Can you work these out from the model? Positions are in its coordinate system, mm. A direction names the side the tool comes from. Round coordinates to 2 decimals unless told otherwise and drop trailing zeros. Loops run counter-clockwise (first coordinate to the right, second up) from the corner with the lowest first, then second, coordinate; pieces in that order, holes last. Notation, with made-up numbers: (-37, 41.25) -> (-15, 41.25) arc R27 ccw to (-15, 78.25) -> close; hole circle Ø8 at (-27, 40). An arc over 180 degrees is marked (long way). Use a Markdown table: item, result.
from build123d import *

# Parameters (mm, degrees)
F0_R      = 1.5
F1_DEPTH  = 1
F2_W      = 1
F2_H      = 30
F3_DEPTH  = 5
F4_W      = 1
F4_H      = 30
F5_DEPTH  = 5
F6_R      = 0.5
F7_DEPTH  = 25
F9_DEPTH  = 25
F10_W     = 5
F10_H     = 35
F11_DEPTH = 25
F12_R     = 1.5
F13_DEPTH = 25


with BuildPart() as f1:
    # F0 (on Right) → F1 (new body)
    with BuildSketch(Plane.YZ):
        with BuildLine():
            Line((-6, 17), (-11, 17))
            Line((-11, 17), (-11, 0))
            Line((-11, 0), (-11, -17))
            Line((-11, -17), (-6, -17))
            Line((-6, -17), (-6, -15))
            Line((-6, -15), (-1.664101, -8.496151))
            ThreePointArc((-1.664101, -8.496151), (0, -7.605551), (1.664101, -8.496151))
            Line((1.664101, -8.496151), (6, -15))
            Line((6, -15), (6, -17))
            Line((6, -17), (11, -17))
            Line((11, -17), (11, 0))
            Line((11, 0), (11, 17))
            Line((11, 17), (6, 17))
            Line((6, 17), (6, 15))
            Line((6, 15), (1.664101, 8.496151))
            ThreePointArc((1.664101, 8.496151), (0, 7.605551), (-1.664101, 8.496151))
            Line((-1.664101, 8.496151), (-6, 15))
            Line((-6, 15), (-6, 17))
        make_face()
        with Locations((-2, 0)):
            Circle(F0_R, mode=Mode.SUBTRACT)
        with Locations((2, 0)):
            Circle(F0_R, mode=Mode.SUBTRACT)
    extrude(amount=F1_DEPTH)

    # F2 (on face) → F3 (join)
    with BuildSketch(Plane.XZ.offset(11)):
        with Locations((0.5, 0)):
            Rectangle(F2_W, F2_H)
    extrude(amount=F3_DEPTH)

    # F4 (on face) → F5 (join)
    with BuildSketch(Plane(origin=(0, 11, 0), x_dir=(-1, 0, 0), z_dir=(0, 1, 0))):
        with Locations((-0.5, 0)):
            Rectangle(F4_W, F4_H)
    extrude(amount=F5_DEPTH)

    # F6 (on face) → F7 (cut)
    with BuildSketch(Plane.YZ.offset(1)):
        with Locations((-11.5, 15)):
            Circle(F6_R)
        with Locations((11.5, 15)):
            Circle(F6_R)
        with Locations((-11.5, -15)):
            Circle(F6_R)
        with Locations((11.5, -15)):
            Circle(F6_R)
    extrude(amount=-F7_DEPTH, mode=Mode.SUBTRACT)

    # F8 (on face) → F9 (cut)
    with BuildSketch(Plane.YZ.offset(1)):
        with BuildLine():
            Line((-7.849001, 2.773501), (-16, 15))
            Line((-16, 15), (-16, -15))
            Line((-16, -15), (-7.849001, -2.773501))
            ThreePointArc((-7.849001, -2.773501), (-7.009252, 0), (-7.849001, 2.773501))
        make_face()
        with BuildLine():
            Line((16, -15), (16, 15))
            Line((16, 15), (7.849001, 2.773501))
            ThreePointArc((7.849001, 2.773501), (7.009252, 0), (7.849001, -2.773501))
            Line((7.849001, -2.773501), (16, -15))
        make_face()
    extrude(amount=-F9_DEPTH, mode=Mode.SUBTRACT)

    # F10 (on face) → F11 (cut)
    with BuildSketch(Plane.YZ.offset(1)):
        with Locations((-17.5, 0)):
            Rectangle(F10_W, F10_H)
        with Locations((17.5, 0)):
            Rectangle(F10_W, F10_H)
    extrude(amount=-F11_DEPTH, mode=Mode.SUBTRACT)

    # F12 (on face) → F13 (cut)
    with BuildSketch(Plane.YZ.offset(1)):
        Circle(F12_R)
        with BuildLine():
            ThreePointArc((-2.447214, -3.605573), (-4.341641, -5.67082), (-1.552786, -5.394427))
            ThreePointArc((-1.552786, -5.394427), (0.341641, -3.32918), (-2.447214, -3.605573))
        make_face()
    extrude(amount=-F13_DEPTH, mode=Mode.SUBTRACT)


solid = f1.part
1. If we mould it in two halves opening along Z, with no side actions, what happens to faces 1 (the cylindrical face through (0.51, 0.36, -3.37)), 2 (the cylindrical face through (0.493, -0.028, -7.606)), 3 (the flat face through (0.5, -15, 14.2))? For each: +Z half, -Z half, draft (parallel to the pull), parting line (faces both ways), or undercut.
Answer sheet:
| item | result |
|---|---|
| face 1 | undercut |
| face 2 | -Z half |
| face 3 | draft |
2. I want a section at C-C (x = 0.8). State how many separate pieces and enclosed holes the cut face has, plus the area to 3 significant figures.
Answer sheet:
| item | result |
|---|---|
| separate pieces | 1 |
| enclosed holes | 2 |
| area | 564 mm² |
3. Will these pins go through, and if not, where does the flat tip stop? pin 1 Ø0.5 at (x, z) = (0.5, -16) entering from +Y; pin 2 Ø0.5 at (x, z) = (0.5, -16) entering from -Y.
Answer sheet:
| item | result |
|---|---|
| pin 1 | stops at y = 11 |
| pin 2 | stops at y = -11 |
4. Which directions (+Z, -Z, +X, -X, +Y, -Y) give clear straight access to the entire face, cutting with the end or side of a thin tool? Please do faces 4 (the flat face through (0.5, 3.8, -11.7)), 5 (the flat face through (0.5, -11, -16)), 6 (the flat face through (0.49, 3.86, 11.79)), 7 (the flat face through (0.5, 11.4, -8.1)).
Answer sheet:
| item | result |
|---|---|
| face 4 | -Z, +X, -X |
| face 5 | -Z, +X, -X, -Y |
| face 6 | +Z, +X, -X |
| face 7 | +X, -X, +Y |
5. I want a section at B-B (z = 0). Please give me the cut outline in (x, y).
Answer sheet:
| item | result |
|---|---|
| outline | (0, -7.01) -> (1, -7.01) -> (1, -3.5) -> (0, -3.5) -> close; (0, 3.5) -> (1, 3.5) -> (1, 7.01) -> (0, 7.01) -> close |
6. I want a section at A-A (y = 3). Please give me the cut outline in (x, z).
Answer sheet:
| item | result |
|---|---|
| outline | (0, -10.5) -> (1, -10.5) -> (1, -1.12) -> (0, -1.12) -> close; (0, 1.12) -> (1, 1.12) -> (1, 10.5) -> (0, 10.5) -> close |
7. I need wall thicknesses on line 1 (Z direction, x = 0.7, y = -0.5); line 2 (Z direction, x = 0.2, y = 14); line 3 (Z direction, x = 0.8, y = -2). Which ranges of each line are inside material? Lowest first, please.
Answer sheet:
| item | result |
|---|---|
| line 1 | z = -7.67 to -5.41, -2.59 to -1.41, 1.41 to 7.67 |
| line 2 | z = -15 to -12, 12 to 15 |
| line 3 | z = -9 to -6.12, -2.88 to -1.5, 1.5 to 9 |
